from build123d import *

# Parameters (mm, degrees)
SKETCH2_R           = 50
BOSS_EXTRUDE1_DEPTH = 20
SKETCH3_R           = 30
BOSS_EXTRUDE2_DEPTH = 30
FILLET1_R           = 2.5
SKETCH4_W           = 110
SKETCH4_H           = 12
CUT_EXTRUDE1_DEPTH  = 10
CUT_EXTRUDE2_REACH  = 88.603


with BuildPart() as part:
    # Sketch2 → Boss-Extrude1 (new body)
    with BuildSketch(Plane.XY):
        Circle(SKETCH2_R)
    extrude(amount=BOSS_EXTRUDE1_DEPTH)

    # Sketch3 → Boss-Extrude2 (add)
    with BuildSketch(Plane.XY.offset(20)):
        Circle(SKETCH3_R)
    extrude(amount=BOSS_EXTRUDE2_DEPTH)

    # Fillet1
    fillet1_edges = [part.edges().sort_by_distance(p)[0] for p in [
        (-30, 0, 20),
    ]]
    fillet(fillet1_edges, radius=FILLET1_R)

    # Sketch4 → Cut-Extrude1 (cut)
    with BuildSketch(Plane(origin=(0, 0, 0), x_dir=(-1, 0, 0), z_dir=(0, 0, -1))):
        Rectangle(SKETCH4_W, SKETCH4_H)
    extrude(amount=-CUT_EXTRUDE1_DEPTH, mode=Mode.SUBTRACT)

    # Cut-Extrude2: up to this face of the body (flat: up to its plane)
    cut_extrude2_end = Plane(part.part.faces().sort_by_distance((0, 24.497956202, 0))[0])
    # Sketch5 → Cut-Extrude2 (cut, up to the picked face)
    with BuildSketch(Plane.XY.offset(50), mode=Mode.PRIVATE) as cut_extrude2_sk1:
        with BuildLine():
            Line((-14.142135624, 5), (-24.142135624, 5))
            Line((-24.142135624, 5), (-24.142135624, -5))
            Line((-24.142135624, -5), (-14.142135624, -5))
            ThreePointArc((-14.142135624, -5), (15, 0), (-14.142135624, 5))
        make_face()
    cut_extrude2_tool1 = split(extrude(cut_extrude2_sk1.sketch, amount=-CUT_EXTRUDE2_REACH, mode=Mode.PRIVATE), bisect_by=cut_extrude2_end, keep=Keep.BOTH, mode=Mode.PRIVATE)
    add(cut_extrude2_tool1.solids().sort_by(Axis((-2.285441, 0, 50), (0, 0, -1)))[0], mode=Mode.SUBTRACT)


solid = part.part
Input: part model. Units: mm. Frame: model coordinates. A direction names the side the tool comes from. Give positions to 0.01 mm unless a question says otherwise; leave off trailing zeros. Loops run counter-clockwise (first coordinate to the right, second up) from the corner with the lowest first, then second, coordinate; pieces in that order, holes last. Notation, with made-up numbers: M 33,-5 L 69,-5 A31 cw 69,25 Z; hole C 87,3.5 d11. An arc over 180 degrees is marked long. Use one line per item in the form item = value.
1. Section query B-B, the plane z = 15. Return the cut outline in (x, y), and give its area (3 significant figures).
Numbers:
outline = C 0,0 d100; hole M -24.14,-5 L -14.14,-5 A15 ccw long -14.14,5 L -24.14,5 Z
area = 7,050 mm²
2. Section query A-A, the plane y = 0. Return the cut outline in (x, z).
Numbers:
outline = M -50,10 L -24.14,10 L -24.14,50 L -30,50 L -30,22.5 A2.5 cw -32.5,20 L -50,20 Z; M 15,10 L 50,10 L 50,20 L 32.5,20 A2.5 cw 30,22.5 L 30,50 L 15,50 Z
3. First-contact query: pin 1 (8 mm diameter, centred on y = 2, z = 33, fed in from +X); pin 2 (6 mm diameter, centred on x = -18.5, z = 16.5, fed in from +Y); pin 3 (3 mm diameter, centred on x = 32.5, z = 6, fed in from -Y). Flat tips, straight axial feed; report the tip coordinate or a pass-through.
Numbers:
pin_1 = 30
pin_2 = 47.54
pin_3 = -39.23
4. Section query D-D, the plane x = -37.5. Return the cut outline in (y, z).
Numbers:
outline = M -33.07,0 L -6,0 L -6,10 L 6,10 L 6,0 L 33.07,0 L 33.07,20 L -33.07,20 Z
5. Line query: L1, parallel to Y at x = 0, z = 19.5; L2, parallel to X at y = 0, z = 18; L3, parallel to Y at x = 0, z = 31. Output: solid intervals per line, ascending.
Numbers:
L1 = -50 to -15, 15 to 50
L2 = -50 to -24.14, 15 to 50
L3 = -30 to -15, 15 to 30
6. Pull-direction query (X, two-part tool) for faces 4 (the face through (6, 14, 50)), 5 (the face through (47.69, 15.02, 9.86)), 6 (the face through (14.99, -0.59, 25.35)); classes: released by +X, released by -X, zero draft, split by the parting line, or undercut.
Numbers:
face_4 = zero draft
face_5 = split by the parting line
face_6 = undercut
7. Section query C-C, the plane x = 0. Return the cut outline in (y, z).
Numbers:
outline = M -50,0 L -15,0 L -15,50 L -30,50 L -30,22.5 A2.5 cw -32.5,20 L -50,20 Z; M 15,0 L 50,0 L 50,20 L 32.5,20 A2.5 cw 30,22.5 L 30,50 L 15,50 Z
8. Reachability of faces 1 (the face through (-19, -5, 30)), 2 (the face through (-29.97, 1.32, 36.06)), 3 (the face through (-31, 6, 5)) from +Z, -Z, +X, -X, +Y, -Y: full face, straight path, thin tool, end or side. Return the list, or none.
Numbers:
face_1 = +Z, -Z
face_2 = +Z
face_3 = -Z, +X, -X
